Part model, mm, in its own coordinate system. A direction names the side the tool comes from. Round coordinates to 2 decimals unless told otherwise and drop trailing zeros. Write each loop counter-clockwise with the first axis right and the second up, starting at its lowest first coordinate (ties: lowest second). Pieces come first, ordered by that corner, then holes. Notation, with made-up numbers: (89, 14.5) -> (128, 14.5) arc R30 cw to (128, 49.5) -> close; hole circle Ø11 at (36.5, 83.25). An arc over 180 degrees is marked (long way). Use CSV: the item, a comma, the result in double quotes. Start each with the question number.
(1) Two-plate mould, pull along Z, no slides. Class faces 6 (the flat face through (-10, 1, 12)), 7 (the flat face through (5, -1, 36)), 8 (the cylindrical face through (5.07, -63.905, 29.867)), 9 (the cylindrical face through (5.07, 56.095, 29.867)): released by +Z, released by -Z, zero draft, split by the parting line, or undercut.
(2) Saw through at A-A (z = 29). Give the cut face in (x, y).
(3) Saw through at B-B (y = 0). Give the cut face in (x, z), plus the area to 3 significant figures.
(4) Saw through at C-C (x = 7). Give the cut face in (y, z).
(5) Probe line 1 (Y direction, x = 0.25, z = 29); line 2 (Y direction, x = 0, z = 5.5); line 3 (Y direction, x = 1, z = 30). List the from-to ranges inside material, lowest first. Write a range as [from, to].
(6) Saw through at D-D (y = 30.5). Give the cut face in (x, z).
(7) Drop flat-ended pins along their axis: pin 1 (1 mm diameter, centred on x = -5, y = -3, fed in from +Z); pin 2 (3 mm diameter, centred on x = 0, z = 2, fed in from +Y); pin 3 (2 mm diameter, centred on y = 16, z = 32, fed in from -X). Give the stop position or say it passes through.
(8) Which spindle directions (+Z, -Z, +X, -X, +Y, -Y) get a long thin tool onto all of the face, cutting with end or side? Do faces 1 (the flat face through (0, 37, 28)), 2 (the cylindrical face through (3.695, -1.532, 19.689)), 3 (the flat face through (3.1, 25, 2)), 4 (the flat face through (-3.1, -25, 2)), 5 (the flat face through (0, 3.1, 2)). Say none if no direction does.
```python
from build123d import *
from build123d.topology import SkipClean

# Parameters (mm, degrees)
EXTRUDE_1_DEPTH      = 14
CUT_EXTRUDE_1_DEPTH  = 44
SKETCH_3_W           = 6.2
SKETCH_3_H           = 6.2
CUT_EXTRUDE_2_DEPTH  = 4
SKETCH_4_R           = 4
CUT_EXTRUDE_3_DEPTH  = 5
SKETCH_5_R           = 2.6
CUT_EXTRUDE_4_DEPTH  = 5
SKETCH_6_W           = 5
SKETCH_6_H           = 44
CUT_EXTRUDE_5_DEPTH  = 10
SKETCH_7_W           = 5
SKETCH_7_H           = 44
CUT_EXTRUDE_6_DEPTH  = 10
EXTRUDE_3_DEPTH      = 48
EXTRUDE_4_DEPTH      = 48
SKETCH_11_W          = 22
SKETCH_11_H          = 140
EXTRUDE_5_DEPTH      = 20
SKETCH_12_R          = 4
CUT_EXTRUDE_7_DEPTH  = 20
SKETCH_13_W          = 10
SKETCH_13_H          = 16
CUT_EXTRUDE_8_DEPTH  = 140
CUT_EXTRUDE_9_DEPTH  = 6
SKETCH_15_R          = 4
CUT_EXTRUDE_10_DEPTH = 20
SKETCH_16_W          = 6.2
SKETCH_16_H          = 22
CUT_EXTRUDE_11_DEPTH = 4


with BuildPart() as part:
    # 草图1 → 凸台-拉伸1 (new body)
    with BuildSketch(Plane.XY):
        Polygon((-15, 22), (-15, -22), (15, -22), (15, 22), (0, 22), align=None)
    extrude(amount=EXTRUDE_1_DEPTH)

    # 草图2 → 切除-拉伸1 (cut)
    with BuildSketch(Plane(origin=(0, 22, 0), x_dir=(1, 0, 0), z_dir=(0, 1, 0))):
        Polygon((-15, 0), (-15, -14), (-10, -4), (-3.1, -4), (-3.1, 0), align=None)
        Polygon((3.1, -4), (10, -4), (15, -14), (15, 0), (3.1, 0), align=None)
    extrude(amount=-CUT_EXTRUDE_1_DEPTH, mode=Mode.SUBTRACT)

    # 草图3 → 切除-拉伸2 (cut)
    with BuildSketch(Plane(origin=(0, 0, 0), x_dir=(-1, 0, 0), z_dir=(0, 0, -1))):
        Rectangle(SKETCH_3_W, SKETCH_3_H)
    extrude(amount=-CUT_EXTRUDE_2_DEPTH, mode=Mode.SUBTRACT)

    # 草图4 → 切除-拉伸3 (cut)
    with BuildSketch(Plane.XY.offset(14)):
        Circle(SKETCH_4_R)
    extrude(amount=-CUT_EXTRUDE_3_DEPTH, mode=Mode.SUBTRACT)

    # 草图5 → 切除-拉伸4 (cut)
    with BuildSketch(Plane.XY.offset(9)):
        Circle(SKETCH_5_R)
    extrude(amount=-CUT_EXTRUDE_4_DEPTH, mode=Mode.SUBTRACT)

    # 草图6 → 切除-拉伸5 (cut)
    with BuildSketch(Plane(origin=(0, 0, 4), x_dir=(-1, 0, 0), z_dir=(0, 0, -1))):
        with Locations((12.5, 0)):
            Rectangle(SKETCH_6_W, SKETCH_6_H)
    extrude(amount=-CUT_EXTRUDE_5_DEPTH, mode=Mode.SUBTRACT)

    # 草图7 → 切除-拉伸6 (cut)
    with BuildSketch(Plane(origin=(0, 0, 4), x_dir=(-1, 0, 0), z_dir=(0, 0, -1))):
        with Locations((-12.5, 0)):
            Rectangle(SKETCH_7_W, SKETCH_7_H)
    extrude(amount=-CUT_EXTRUDE_6_DEPTH, mode=Mode.SUBTRACT)

    # 草图9 → 凸台-拉伸3 (add)
    with BuildSketch(Plane(origin=(0, 22, 0), x_dir=(1, 0, 0), z_dir=(0, 1, 0))):
        Polygon((-3.1, 0), (3.1, 0), (3.1, -4), (10, -4), (10, -14), (-10, -14), (-10, -4), (-3.1, -4), align=None)
    extrude(amount=EXTRUDE_3_DEPTH)

    # 草图10 → 凸台-拉伸4 (add)
    with BuildSketch(Plane(origin=(0, -22, 0), x_dir=(-1, 0, 0), z_dir=(0, -1, 0))):
        Polygon((10, -14), (-10, -14), (-10, -4), (-3.1, -4), (-3.1, 0), (3.1, 0), (3.1, -4), (10, -4), align=None)
    extrude(amount=EXTRUDE_4_DEPTH)

    # 草图11 → 凸台-拉伸5 (add)
    with BuildSketch(Plane(origin=(10, 0, 0), x_dir=(0, 0, -1), z_dir=(1, 0, 0))):
        with Locations((-25, 0)):
            Rectangle(SKETCH_11_W, SKETCH_11_H)
    extrude(amount=-EXTRUDE_5_DEPTH)

    # 草图12 → 切除-拉伸7 (cut)
    with BuildSketch(Plane(origin=(10, 0, 0), x_dir=(0, 0, -1), z_dir=(1, 0, 0))):
        with Locations((-29, 60)):
            Circle(SKETCH_12_R)
        with Locations((-29, -60)):
            Circle(SKETCH_12_R)
    extrude(amount=-CUT_EXTRUDE_7_DEPTH, mode=Mode.SUBTRACT)

    # 草图13 → 切除-拉伸8 (cut)
    with BuildSketch(Plane.XZ.offset(70)):
        with Locations((-5, 28)):
            Rectangle(SKETCH_13_W, SKETCH_13_H)
    extrude(amount=-CUT_EXTRUDE_8_DEPTH, mode=Mode.SUBTRACT)

    # 草图14 → 切除-拉伸9 (cut)
    with BuildSketch(Plane.XY.offset(20)):
        with BuildLine():
            ThreePointArc((4, 0), (2.828427125, 2.828427125), (0, 4))
            Line((0, 4), (0, -4))
            ThreePointArc((0, -4), (2.828427125, -2.828427125), (4, 0))
        make_face()
        with BuildLine():
            Line((0, -4), (0, 4))
            ThreePointArc((0, 4), (-4, 0), (0, -4))
        make_face()
    extrude(amount=-CUT_EXTRUDE_9_DEPTH, mode=Mode.SUBTRACT)

    # 草图15 → 切除-拉伸10 (cut)
    with SkipClean():  # the faces are left unmerged after this step: merging them gives an invalid solid
        with BuildSketch(Plane.XY.offset(36)):
            Circle(SKETCH_15_R)
        extrude(amount=-CUT_EXTRUDE_10_DEPTH, mode=Mode.SUBTRACT)

    # 草图16 → 切除-拉伸11 (cut)
    with SkipClean():  # the faces are left unmerged after this step: merging them gives an invalid solid
        with BuildSketch(Plane(origin=(0, 0, 0), x_dir=(-1, 0, 0), z_dir=(0, 0, -1))):
            with Locations((0, 59)):
                Rectangle(SKETCH_16_W, SKETCH_16_H)
            with Locations((0, -59)):
                Rectangle(SKETCH_16_W, SKETCH_16_H)
        extrude(amount=-CUT_EXTRUDE_11_DEPTH, mode=Mode.SUBTRACT)


solid = part.part
```
Answers:
1,face 6,"zero draft"
1,face 7,"released by +Z"
1,face 8,"undercut"
1,face 9,"undercut"
2,outline,"(0, -70) -> (10, -70) -> (10, -64) -> (0, -64) -> close; (0, -56) -> (10, -56) -> (10, 56) -> (0, 56) -> (0, 4) arc R4 cw to (0, -4) -> close; (0, 64) -> (10, 64) -> (10, 70) -> (0, 70) -> close"
3,outline,"(-10, 4) -> (-2.6, 4) -> (-2.6, 9) -> (-4, 9) -> (-4, 20) -> (-10, 20) -> close; (2.6, 4) -> (10, 4) -> (10, 36) -> (4, 36) -> (4, 9) -> (2.6, 9) -> close"
3,area,"302 mm²"
4,outline,"(-70, 4) -> (70, 4) -> (70, 36) -> (-70, 36) -> close; hole circle Ø8 at (-60, 29); hole circle Ø8 at (60, 29)"
5,line 1,"y = [-70, -64], [-56, -3.99], [3.99, 56], [64, 70]"
5,line 2,"y = [-70, -2.6], [2.6, 70]"
5,line 3,"y = [-70, -63.87], [-56.13, -3.87], [3.87, 56.13], [63.87, 70]"
6,outline,"(-10, 4) -> (-3.1, 4) -> (-3.1, 0) -> (3.1, 0) -> (3.1, 4) -> (10, 4) -> (10, 36) -> (0, 36) -> (0, 20) -> (-10, 20) -> close"
7,pin 1,"stops at z = 20"
7,pin 2,"stops at y = 48"
7,pin 3,"stops at x = 0"
8,face 1,"+Z, -X, +Y, -Y"
8,face 2,"+Z"
8,face 3,"-Z, +X, +Y, -Y"
8,face 4,"-Z, -X, +Y, -Y"
8,face 5,"-Z, +X, -X"
